from build123d import *

# Parameters (mm, degrees)
SKETCH1_R                      = 18
BOSS_EXTRUDE1_DEPTH            = 8
SKETCH2_R                      = 22.5
BOSS_EXTRUDE2_DEPTH            = 8
CHAMFER1_SIZE                  = 0.5
SKETCH3_R                      = 7.5
CUT_EXTRUDE1_DEPTH             = 36.616007637
CBORE_FOR_M5_SHCS1_D           = 5.5
CBORE_FOR_M5_SHCS1_CBORE_D     = 9
CBORE_FOR_M5_SHCS1_CBORE_DEPTH = 5
CIRPATTERN1_COUNT              = 4


with BuildPart() as part:
    # Sketch1 → Boss-Extrude1 (new body)
    with BuildSketch(Plane.XY):
        Circle(SKETCH1_R)
    extrude(amount=BOSS_EXTRUDE1_DEPTH)

    # Sketch2 → Boss-Extrude2 (add)
    with BuildSketch(Plane(origin=(0, 0, 0), x_dir=(-1, 0, 0), z_dir=(0, 0, -1))):
        Circle(SKETCH2_R)
    extrude(amount=BOSS_EXTRUDE2_DEPTH)

    # Chamfer1
    chamfer1_edges = [part.edges().sort_by_distance(p)[0] for p in [
        (-18, 0, 8),
        (22.5, 0, 0),
        (22.5, 0, -8),
    ]]
    chamfer(chamfer1_edges, length=CHAMFER1_SIZE)

    # Sketch3 → Cut-Extrude1 (cut, through all)
    with BuildSketch(Plane(origin=(0, 0, -8), x_dir=(-1, 0, 0), z_dir=(0, 0, -1))):
        Circle(SKETCH3_R)
    extrude(amount=-CUT_EXTRUDE1_DEPTH, mode=Mode.SUBTRACT)

    # CBORE for M5 SHCS1 (through all)
    with Locations(Plane(origin=(0, 0, -8), x_dir=(-1, 0, 0), z_dir=(0, 0, -1))):
        with Locations((0, 13)):
            cbore_for_m5_shcs1 = CounterBoreHole(CBORE_FOR_M5_SHCS1_D / 2, CBORE_FOR_M5_SHCS1_CBORE_D / 2, CBORE_FOR_M5_SHCS1_CBORE_DEPTH)

    # CirPattern1: CBORE for M5 SHCS1 ×4 about axis
    cirpattern1_axis = Axis((0, 0, 0), (0, 0, 1))
    for i in range(1, CIRPATTERN1_COUNT):
        add(cbore_for_m5_shcs1.rotate(cirpattern1_axis, i * 360 / CIRPATTERN1_COUNT), mode=Mode.SUBTRACT)


solid = part.part
Read the model definition and answer for the solid it produces. Units are mm, in the model's axes. A direction names the side the tool comes from. Round coordinates to 2 decimals unless told otherwise and drop trailing zeros. Loops run counter-clockwise (first coordinate to the right, second up) from the corner with the lowest first, then second, coordinate; pieces in that order, holes last.
Q1. Determine the mould class of faces 4 (the face through (8.3, -16.2, 0)), 5 (the face through (-10.382, -19.961, -3.951)), 6 (the face through (-0.358, 15.727, 2.577)) for opening direction X: released by +X, released by -X, zero draft, split by the parting line, or undercut.
Q2. Which of the six approach directions +Z, -Z, +X, -X, +Y, -Y give full straight-line access (tool end or side, diameter ignored) to faces 1 (the face through (-2.343, 17.847, 3.698)), 2 (the face through (10, 0, -3)), 3 (the face through (15.727, 0.358, 2.577))?
Q3. Section C-C on z = 4 is taken. Write down the section's boundary in (x, y), and give its area (3 significant figures).
Q4. Section B-B on z = -5.5 is taken. Write down the section's boundary in (x, y).
Q5. Each of these flat-tipped pins is pushed along its axis until it touches: pin 1 (13.5 mm diameter, centred on x = 0, y = 0, fed in from +Z); pin 2 (5 mm diameter, centred on y = -7.5, z = -0.5, fed in from -X); pin 3 (7 mm diameter, centred on x = 13, y = 0, fed in from -Z); pin 4 (1 mm diameter, centred on y = -1, z = -1.5, fed in from +X). Where does it stop, or does it pass through?
Q6. Consider probe 1 along Y at (x, z) = (0, 4); probe 2 along Y at (x, z) = (0, -2.75); probe 3 along X at (y, z) = (1.5, 6.5). Determine where each line is inside the solid, lowest interval first.
Q7. Section A-A on x = 0 is taken. Give the number of separate pieces and of enclosed holes in the cut face, and give its area (3 significant figures).
Output:
1. face 4: zero draft
1. face 5: split by the parting line
1. face 6: undercut
2. face 1: +Z
2. face 2: -Z
2. face 3: +Z, -Z
3. outline: circle Ø36 at (0, 0); hole circle Ø5.5 at (-13, 0); hole circle Ø15 at (0, 0); hole circle Ø5.5 at (0, -13); hole circle Ø5.5 at (0, 13); hole circle Ø5.5 at (13, 0)
3. area: 746 mm2
4. outline: circle Ø45 at (0, 0); hole circle Ø9 at (-13, 0); hole circle Ø15 at (0, 0); hole circle Ø9 at (0, -13); hole circle Ø9 at (0, 13); hole circle Ø9 at (13, 0)
5. pin 1: passes through
5. pin 2: stops at x = -21.94
5. pin 3: stops at z = -3
5. pin 4: stops at x = 22.49
6. probe 1: y = -18 to -15.75, -10.25 to -7.5, 7.5 to 10.25, 15.75 to 18
6. probe 2: y = -22.5 to -15.75, -10.25 to -7.5, 7.5 to 10.25, 15.75 to 22.5
6. probe 3: x = -17.94 to -15.3, -10.7 to -7.35, 7.35 to 10.7, 15.3 to 17.94
7. separate pieces: 4
7. enclosed holes: 0
7. area: 196 mm2
